Build history of the part. All positions in model axes, mm. A direction names the side the tool comes from. Give positions to 0.01 mm unless a question says otherwise; leave off trailing zeros. Write each loop counter-clockwise with the first axis right and the second up, starting at its lowest first coordinate (ties: lowest second). Pieces come first, ordered by that corner, then holes. Notation, with made-up numbers: (17, 22.5) -> (65, 22.5) arc R13 ccw to (65, 31.5) -> close; hole circle Ø6 at (59.25, 16). An arc over 180 degrees is marked (long way). One line per question, with ' | ' between items. Start each with the question number.
(1) Tool access for faces 4 (the flat face through (-11, -150, -49)), 5 (the cylindrical face through (-18.98, -0.84, 52.19)): list every direction of +Z, -Z, +X, -X, +Y, -Y with a clear straight run to the whole face (end or side of a thin tool).
(2) Band-saw the part on B-B, the plane x = 0. Count the separate pieces of the cut face and the enclosed holes in it, and give its area (3 significant figures).
(3) Pull direction X, two halves, no side cores. Call faces 1 (the cylindrical face through (-27.31, -2.1, -42.835)), 2 (the cylindrical face through (-22.887, 2.1, -44.004)), 3 (the flat face through (6, 17, 55)): released by +X, released by -X, zero draft, split by the parting line, or undercut.
(4) Band-saw the part on D-D, the plane y = 123. Give the cut face in (x, z).
(5) Pin check, flat tips, straight feed: P1, Ø1, axis at x = 25.5, y = 84.5, coming from the -Z side; P2, Ø8, axis at y = 47, z = 9, coming from the -X side; P3, Ø3, axis at y = -60, z = -20, coming from the -X side. Stop position of each tip, or through.
(6) Band-saw the part on A-A, the plane z = 0. Give the cut face in (x, y).
(7) Band-saw the part on C-C, the plane x = 43. Give the cut face in (y, z), and give its area (3 significant figures).
(8) Drill centre lines: probe 1 along X at (y, z) = (0, 53); probe 2 along Z at (x, y) = (0, 37); probe 3 along Z at (x, y) = (-15, 19). Where is each one in solid material? Low to high. Write a range as from..to.
Autodesk Inventor part; units mm, degrees
ref_plane "YZ Plane" through (0, 0, 0) normal (1, 0, 0) x (0, 1, 0)
ref_plane "XZ Plane" through (0, 0, 0) normal (0, 1, 0) x (-1, 0, 0)
ref_plane "XY Plane" through (0, 0, 0) normal (0, 0, 1) x (1, 0, 0)
sketch "Szkic8" plane through (0, 0, 0) normal (0, 1, 0) x (-1, 0, 0)
  circle A0 centre (0, 0) radius 50.8
  circle A1 centre (0, 0) radius 49.6
  dimension "d53" = 101.6
  dimension "d54" = 1.2
extrude "Wyciągnięcie proste2" add sketch "Szkic8" along normal mid plane 300
sketch "Szkic13" plane through (0, 0, 0) normal (0, 0, 1) x (1, 0, 0)
  circle A0 centre (0, 0) radius 19
  circle A1 centre (0, 0) radius 17.8
  dimension "d67" = 38
  dimension "d68" = 1.2
extrude "Wyciągnięcie proste6" add sketch "Szkic13" along normal blind 55
sketch "Szkic14" plane through (0, 0, 55) normal (0, 0, 1) x (1, 0, 0)
  circle A0 centre (0, 0) radius 17.8
extrude "Wyciągnięcie proste7" cut sketch "Szkic14" against normal blind 55
sketch "Szkic15" plane through (0, -150, 0) normal (0, -1, 0) x (1, 0, 0)
  circle A0 centre (0, 0) radius 49.6
extrude "Wyciągnięcie proste8" cut sketch "Szkic15" against normal blind 300
fillet "Zaokrąglenie3" radius 1.2 2 edges at (-0.0019, 19, 50.8) (-0.0001, -19, 50.8)
fillet "Zaokrąglenie4" radius 2.4 2 edges at (-0.0005, -17.8, 49.6) (-0.001, 17.8, 49.6)
equation "\"d53\" = OD"
equation "\"d54\" = THK"
equation "\"d55\" = L1"
equation "\"d67\" = OD2"
equation "\"d68\" = THK"
equation "\"d69\" = L2"
equation "\"d71\" = L2"
equation "\"d73\" = L1"
equation "\"d75\" = THK"
equation "\"d76\" = 2 * THK"
equation "\"SzerokośćGięciaPodcięcia\" = Grubość"
equation "\"RozmiarPodcięciaNarożnika\" = 4 * Grubość"
equation "\"PromieńPrzejścia\" = PromieńGięcia"
equation "\"Rozmiar_promienia_Jacobiego\" = PromieńGięcia"
equation "\"Wielk_odstępu\" = Grubość"
equation "\"d2\" = PromieńGięcia"
equation "\"d23\" = PromieńGięcia"
equation "\"OD\" = 101.6"
equation "\"THK\" = 1.2"
equation "\"L1\" = 300"
equation "\"L2\" = 55"
equation "\"OD2\" = 38"
properties part number "Trójnik red. krótki  Ø101,6 38 101,6 s=1,2 L=300" material "304"
Results:
1) face 4: +Z, -Z, +X, -X, -Y | face 5: +Z
2) separate pieces: 3 | enclosed holes: 0 | area: 686 mm²
3) face 1: split by the parting line | face 2: undercut | face 3: zero draft
4) outline: circle Ø101.6 at (0, 0); hole circle Ø99.2 at (0, 0)
5) P1: stops at z = -44.22 | P2: stops at x = -50.55 | P3: stops at x = -47.31
6) outline: (-50.8, -150) -> (-49.6, -150) -> (-49.6, 150) -> (-50.8, 150) -> close; (49.6, -150) -> (50.8, -150) -> (50.8, 150) -> (49.6, 150) -> close
7) outline: (-150, -27.05) -> (150, -27.05) -> (150, -24.72) -> (-150, -24.72) -> close; (-150, 24.72) -> (150, 24.72) -> (150, 27.05) -> (-150, 27.05) -> close | area: 1,400 mm²
8) probe 1: x = -19..-17.8, 17.8..19 | probe 2: z = -50.8..-49.6, 49.6..50.8 | probe 3: z = -48.53..-47.28, 47.28..48.53
